Part print with two shaded views. Sizes in mm from the minimum x, y, z corner. Give positions to 0.01 mm unless a question says otherwise; leave off trailing zeros. Loops run counter-clockwise (first coordinate to the right, second up) from the corner with the lowest first, then second, coordinate; pieces in that order, holes last. Notation, with made-up numbers: M 52.5,11 L 91.5,11 A23 cw 91.5,20 Z; hole C 61,-2.75 d3. An arc over 180 degrees is marked long. Answer as a JSON object with one key per item and string values. Group by question number.
1. Slice it at A-A (y = 3.5). List the corners of the cut face in (x, z), then the cut area to 3 significant figures.
2. Mould opens along Y. For the marked faces 1, 2 and 3 say: released by +Y, released by -Y, zero draft, split by the parting line, or undercut.
3. Drill centre lines: line 1 along Y through (x, z) = (3.5, 1.1); line 2 along X through (y, z) = (4, 2.15); line 3 along X through (y, z) = (3.25, 1.2). Where is each one in solid material? Low to high. Write a range as [from, to].
4. Slice it at D-D (z = 2.4). List the corners of the cut face in (x, y), then the cut area to 3 significant figures.
5. Slice it at C-C (z = 0.2). List the corners of the cut face in (x, y), then the cut area to 3 significant figures.
6. Drop flat-ended pins along their axis: pin 1 Ø3.5 at (x, y) = (3.5, 3.5) entering from -Z; pin 2 Ø1 at (x, y) = (5, 4) entering from +Z. Give the stop position or say it passes through.
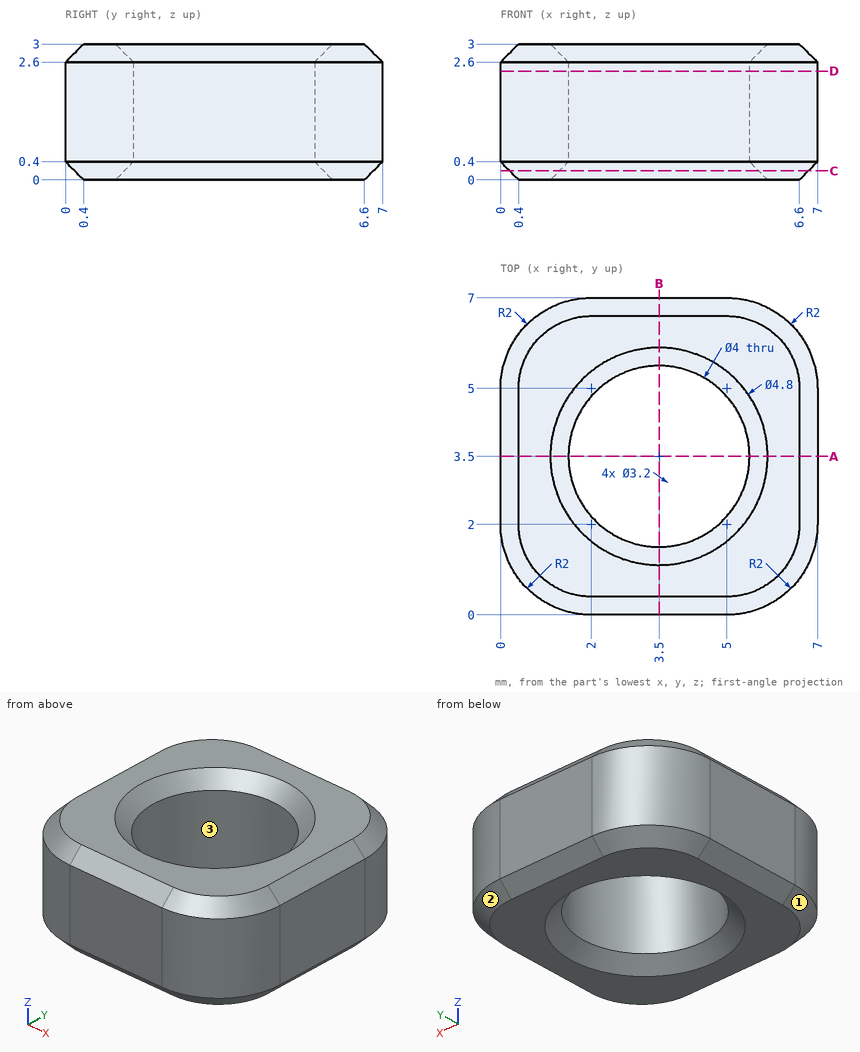
Established:
{
 "1": {"outline": "M 0,0.4 L 0.4,0 L 1.1,0 L 1.5,0.4 L 1.5,2.6 L 1.1,3 L 0.4,3 L 0,2.6 Z; M 5.5,0.4 L 5.9,0 L 6.6,0 L 7,0.4 L 7,2.6 L 6.6,3 L 5.9,3 L 5.5,2.6 Z", "area": "8.36 mm^2"},
 "2": {"face 1": "released by -Y", "face 2": "released by +Y", "face 3": "undercut"},
 "3": {"line 1": "y = [0, 1.5], [5.5, 7]", "line 2": "x = [0, 1.56], [5.44, 7]", "line 3": "x = [0, 1.52], [5.48, 7]"},
 "4": {"outline": "M 0,2 A2 ccw 2,0 L 5,0 A2 ccw 7,2 L 7,5 A2 ccw 5,7 L 2,7 A2 ccw 0,5 Z; hole C 3.5,3.5 d4", "area": "33.0 mm^2"},
 "5": {"outline": "M 0.2,2 A1.8 ccw 2,0.2 L 5,0.2 A1.8 ccw 6.8,2 L 6.8,5 A1.8 ccw 5,6.8 L 2,6.8 A1.8 ccw 0.2,5 Z; hole C 3.5,3.5 d4.4", "area": "25.6 mm^2"},
 "6": {"pin 1": "passes through", "pin 2": "stops at z = 2.68"}
}
